from build123d import *

# Parameters (mm, degrees)
SKETCH2_R           = 2.0828
BOSS_EXTRUDE1_DEPTH = 3.175


with BuildPart() as part:
    # Sketch2 → Boss-Extrude1 (new body)
    with BuildSketch(Plane(origin=(0, 0, 0), x_dir=(1, 0, 0), z_dir=(0, 1, 0))):
        Polygon((3.175, 13.229166667), (3.175, 25.929166667), (0, 25.929166667), (0, 38.629166667), (3.175, 38.629166667), (3.175, 51.329166667), (0, 51.329166667), (0, 64.029166667), (3.175, 64.029166667), (3.175, 76.729166667), (0, 76.729166667), (0, 89.429166667), (3.175, 89.429166667), (3.175, 102.129166667), (142.875, 102.129166667), (142.875, 89.429166667), (146.05, 89.429166667), (146.05, 76.729166667), (142.875, 76.729166667), (142.875, 64.029166667), (146.05, 64.029166667), (146.05, 51.329166667), (142.875, 51.329166667), (142.875, 38.629166667), (146.05, 38.629166667), (146.05, 25.929166667), (142.875, 25.929166667), (142.875, 13.229166667), (146.05, 13.229166667), (146.05, 0.529166667), (0, 0.529166667), (0, 13.229166667), align=None)
        with Locations(Location((136.525, 57.679166667, 0), (0, 0, 90))):
            Circle(SKETCH2_R, mode=Mode.SUBTRACT)
        with Locations(Location((9.525, 13.229166667, 0), (0, 0, 270))):
            Circle(SKETCH2_R, mode=Mode.SUBTRACT)
        with Locations(Location((9.525, 57.679166667, 0), (0, 0, 270))):
            Circle(SKETCH2_R, mode=Mode.SUBTRACT)
        with Locations(Location((136.525, 13.229166667, 0), (0, 0, 90))):
            Circle(SKETCH2_R, mode=Mode.SUBTRACT)
        with Locations(Location((79.375, 6.879166667, 0), (0, 0, 270))):
            Circle(SKETCH2_R, mode=Mode.SUBTRACT)
        with Locations(Location((73.025, 13.229166667, 0), (0, 0, 270))):
            Circle(SKETCH2_R, mode=Mode.SUBTRACT)
        with Locations(Location((66.675, 6.879166667, 0), (0, 0, 270))):
            Circle(SKETCH2_R, mode=Mode.SUBTRACT)
        with Locations(Location((117.475, 95.779166667, 0), (0, 0, 270))):
            Circle(SKETCH2_R, mode=Mode.SUBTRACT)
        with Locations(Location((28.575, 95.779166667, 0), (0, 0, 90))):
            Circle(SKETCH2_R, mode=Mode.SUBTRACT)
    extrude(amount=BOSS_EXTRUDE1_DEPTH)


solid = part.part
Input: part model. Units: mm. Frame: model coordinates. A direction names the side the tool comes from. Coordinates: 2 decimals unless noted, no trailing zeros. Order: outer loops, then holes, each group sorted by start corner. A loop starts at its lowest first (then second) coordinate and runs counter-clockwise, first axis right, second up. Notation, with made-up numbers: M 32.25,74.25 L 62.25,74.25 A22 ccw 62.25,107.25 Z; hole C 52.5,10 d1. An arc over 180 degrees is marked long. Write item = value, one per line. Start each with the question number.
(1) Line query: line 1 along X through (y, z) = (2.35, -95.5) (3 decimals); line 2 along X through (y, z) = (1.55, -12); line 3 along X through (y, z) = (2.65, -14) (3 decimals). Output: solid intervals per line, ascending. Write a range as [from, to].
(2) Section B-B on z = -48.5. Output: boundary loops of the cut face in (x, y) (3 decimals).
(3) Section A-A on y = 2.35. Give the number of separate pieces and of enclosed holes in the cut face, and give its area (3 significant figures).
(4) Reachability of faces 1 (the flat face through (3.175, 2, -45)), 2 (the flat face through (74, 3.175, -52)), 3 (the flat face through (144, 2, -76.729)), 4 (the flat face through (3.175, 2, -96)), 5 (the flat face through (144, 2, -89.429)) from +Z, -Z, +X, -X, +Y, -Y: full face, straight path, thin tool, end or side. Return the list, or none.
(5) First-contact query: P1, Ø6, axis at x = 118, z = -50, coming from the -Y side; P2, Ø1.6, axis at y = 1, z = -68, coming from the +X side (3 decimals); P3, Ø3.5, axis at x = 66.68, z = -6.88, coming from the +Y side; P4, Ø1, axis at y = 1.5, z = -67.5, coming from the -X side (3 decimals). Flat tips, straight axial feed; report the tip coordinate or a pass-through.
Result set:
q1.line_1 = [3.175, 26.511], [30.639, 115.411], [119.539, 142.875]
q1.line_2 = [0, 7.84], [11.21, 71.34], [74.71, 134.84], [138.21, 146.05]
q1.line_3 = [3.175, 7.59], [11.46, 71.09], [74.96, 134.59], [138.46, 142.875]
q2.outline = M 3.175,0 L 142.875,0 L 142.875,3.175 L 3.175,3.175 Z
q3.separate_pieces = 1
q3.enclosed_holes = 9
q3.area = 14,400 mm²
q4.face_1 = -X, +Y, -Y
q4.face_2 = +Z, -Z, +X, -X, +Y
q4.face_3 = +X, +Y, -Y
q4.face_4 = -Z, -X, +Y, -Y
q4.face_5 = -Z, +X, +Y, -Y
q5.P1 = 0
q5.P2 = 142.875
q5.P3 = through
q5.P4 = 3.175
